CAD build for the part. Positions are in the model's coordinates, mm. A direction names the side the tool comes from. Round coordinates to 2 decimals unless told otherwise and drop trailing zeros. Loops run counter-clockwise (first coordinate to the right, second up) from the corner with the lowest first, then second, coordinate; pieces in that order, holes last. Notation, with made-up numbers: M 64.25,25 L 109.25,25 A23 cw 109.25,46 Z; hole C -26.75,85 d6. An arc over 180 degrees is marked long. Put each result on its own line as item: value. Start each with the question number.
from build123d import *

# Parameters (mm, degrees)
SKETCH_1_W          = 34
SKETCH_1_H          = 34
EXTRUDE_1_DEPTH     = 23.5
SKETCH_2_W          = 7.807367758
SKETCH_2_H          = 1.293413098
SKETCH_2_W_2        = 1.293413098
SKETCH_2_H_2        = 7.807367758
CUT_EXTRUDE_1_DEPTH = 53.792044855
CUT_EXTRUDE_2_DEPTH = 53.792044855
SKETCH_4_W          = 2
SKETCH_4_H          = 8.049048512
EXTRUDE_2_DEPTH     = 47
M5X0_8_1_D          = 4.2
M5X0_8_1_DEPTH      = 12.4
M5X0_8_1_TIP        = 1.2618073
SKETCH_7_R          = 4
EXTRUDE_3_DEPTH     = 18
EXTRUDE_START       = 8
SKETCH_8_R          = 4
EXTRUDE_4_DEPTH     = 8
M4X0_7_1_D          = 3.3
M4X0_7_1_DEPTH      = 10.1
M4X0_7_1_TIP        = 0.991420021
M5X0_8_2_D          = 4.2
M5X0_8_2_DEPTH      = 12.4
M5X0_8_2_TIP        = 1.2618073
CHAMFER_1_SIZE      = 0.5


with BuildPart() as part:
    # 草图1 → 凸台-拉伸1 (new, symmetric)
    with BuildSketch(Plane(origin=(0, 0, 0), x_dir=(0, 0, -1), z_dir=(1, 0, 0))):
        Rectangle(SKETCH_1_W, SKETCH_1_H)
    extrude(amount=EXTRUDE_1_DEPTH, both=True)

    # 草图2 → 切除-拉伸1 (cut, through all)
    with BuildSketch(Plane(origin=(23.5, 0, 0), x_dir=(0, 0, -1), z_dir=(1, 0, 0))):
        with Locations((0, 16.353293451)):
            Rectangle(SKETCH_2_W, SKETCH_2_H)
        with Locations((0, -16.353293451)):
            Rectangle(SKETCH_2_W, SKETCH_2_H)
        with Locations((16.353293451, 0)):
            Rectangle(SKETCH_2_W_2, SKETCH_2_H_2)
    extrude(amount=-CUT_EXTRUDE_1_DEPTH, mode=Mode.SUBTRACT)

    # 草图3 → 切除-拉伸2 (cut, through all)
    with BuildSketch(Plane(origin=(23.5, 0, 0), x_dir=(0, 0, -1), z_dir=(1, 0, 0))):
        Polygon((-17, 8.160891433), (-14.681905921, 8.160891433), (-12.449444795, 5.490864716), (-15.849248052, 2.648223271), (-17, 4.024524256), align=None)
        Polygon((-17, -4.024524256), (-17, -8.160891433), (-14.681905921, -8.160891433), (-12.449444795, -5.490864716), (-15.849248052, -2.648223271), align=None)
    extrude(amount=-CUT_EXTRUDE_2_DEPTH, mode=Mode.SUBTRACT)

    # 草图4 → 凸台-拉伸2 (add)
    with BuildSketch(Plane(origin=(23.5, 0, 0), x_dir=(0, 0, -1), z_dir=(1, 0, 0))):
        with Locations((-18, 0)):
            Rectangle(SKETCH_4_W, SKETCH_4_H)
    extrude(amount=-EXTRUDE_2_DEPTH)

    # M5x0.8 螺纹孔1
    with Locations(Plane.XY.offset(19)):
        with Locations((14.396569206, 0)):
            Hole(M5X0_8_1_D / 2, depth=M5X0_8_1_DEPTH)
            with Locations((0, 0, -(M5X0_8_1_DEPTH + M5X0_8_1_TIP / 2))):  # 118° drill point
                Cone(0, M5X0_8_1_D / 2, M5X0_8_1_TIP, mode=Mode.SUBTRACT)

    # 草图7 → 凸台-拉伸3 (add)
    with BuildSketch(Plane(origin=(23.5, 0, 0), x_dir=(0, 0, -1), z_dir=(1, 0, 0))):
        Circle(SKETCH_7_R)
    extrude(amount=EXTRUDE_3_DEPTH)

    # 草图8 → 凸台-拉伸4 (add)
    with BuildSketch(Plane.ZY.offset(23.5).offset(EXTRUDE_START)):
        with Locations(Location((0, 0, 0), (0, 0, 180))):
            Circle(SKETCH_8_R)
    extrude(amount=-EXTRUDE_4_DEPTH)

    # M4x0.7 螺纹孔1
    with Locations(Plane.ZY.offset(31.5)):
        with Locations((0, 0)):
            Hole(M4X0_7_1_D / 2, depth=M4X0_7_1_DEPTH)
            with Locations((0, 0, -(M4X0_7_1_DEPTH + M4X0_7_1_TIP / 2))):  # 118° drill point
                Cone(0, M4X0_7_1_D / 2, M4X0_7_1_TIP, mode=Mode.SUBTRACT)

    # M5x0.8 螺纹孔2
    with Locations(Plane(origin=(23.5, 0, 0), x_dir=(0, 0, -1), z_dir=(1, 0, 0))):
        with Locations((-12, 12), (12, 12), (12, -12), (-12, -12)):
            Hole(M5X0_8_2_D / 2, depth=M5X0_8_2_DEPTH)
            with Locations((0, 0, -(M5X0_8_2_DEPTH + M5X0_8_2_TIP / 2))):  # 118° drill point
                Cone(0, M5X0_8_2_D / 2, M5X0_8_2_TIP, mode=Mode.SUBTRACT)

    # 倒角1
    chamfer_1_edges = [part.edges().sort_by_distance(p)[0] for p in [
        (41.5, 0, 4),
    ]]
    chamfer(chamfer_1_edges, length=CHAMFER_1_SIZE)


solid = part.part
(1) Drill centre lines: line 1 along Y through (x, z) = (18.75, 12); line 2 along Y through (x, z) = (14.25, 12). Where is each one in solid material? Low to high.
(2) Cut at A-A on x = -6.5. List the corners of the cut face in (y, z), and give its area (3 significant figures).
(3) Mould opens along Y. For faces 5 (the conical face through (-20.6, -0.1, 0.3)), 6 (the cylindrical face through (-27.556, 3.905, 0.867)), 7 (the flat face through (0.33, -6.84, 13.58)), 8 (the flat face through (0, -4.025, 18)) say: +Y half, -Y half, draft (parallel to the pull), parting line (faces both ways), or undercut.
(4) Flat gauge pins, fed straight in: pin 1 Ø4 at (y, z) = (-7.5, -0.5) entering from -X; pin 2 Ø0.6 at (x, y) = (10, 16.5) entering from +Z; pin 3 Ø3.5 at (x, y) = (14.4, 0) entering from +Z. Where does each tip first touch, or does it go through?
(5) Tool access for faces 1 (the flat face through (0, 0, -15.707)), 2 (the flat face through (0.329, -4.089, 14.126)), 3 (the flat face through (0, -8.161, 16)), 4 (the cylindrical face through (17.21, 12.09, 9.9)): list every direction of +Z, -Z, +X, -X, +Y, -Y with a clear straight run to the whole face (end or side of a thin tool).
Taken from the geometry:
1. line 1: -17 to -14.1, -9.9 to 9.9, 14.1 to 17
1. line 2: -17 to -14.1, -9.9 to -2.09, 2.09 to 9.9, 14.1 to 17
2. outline: M -17,-17 L -3.9,-17 L -3.9,-15.71 L 3.9,-15.71 L 3.9,-17 L 17,-17 L 17,-3.9 L 15.71,-3.9 L 15.71,3.9 L 17,3.9 L 17,17 L 8.16,17 L 8.16,14.68 L 5.49,12.45 L 2.65,15.85 L 4.02,17 L 4.02,19 L -4.02,19 L -4.02,17 L -2.65,15.85 L -5.49,12.45 L -8.16,14.68 L -8.16,17 L -17,17 L -17,3.9 L -15.71,3.9 L -15.71,-3.9 L -17,-3.9 Z
2. area: 1,110 mm2
3. face 5: undercut
3. face 6: parting line
3. face 7: undercut
3. face 8: -Y half
4. pin 1: x = -23.5
4. pin 2: z = 17
4. pin 3: z = 6.39
5. face 1: -Z, +X, -X
5. face 2: +X, -X
5. face 3: +Z, +X, -X
5. face 4: +X
